```python
from build123d import *

# Parameters (mm, degrees)
F1_DEPTH = 1.06
F3_DEPTH = 1.06
F5_DEPTH = 3
F7_DEPTH = 25
F9_DEPTH = 3.6


with BuildPart() as f1:
    # F0 (on Top) → F1 (new body)
    with BuildSketch(Plane.XY):
        with BuildLine():
            ThreePointArc((-41, -6.825), (-39.256131, -8.181908), (-37.1, -8.665))
            Line((-37.1, -8.665), (-0.75, -8.665))
            ThreePointArc((-0.75, -8.665), (-0.21967, -8.44533), (0, -7.915))
            Line((0, -7.915), (0, 0))
            ThreePointArc((0, 0), (0.294358, 0.710642), (1.005, 1.005))
            Line((1.005, 1.005), (3.39, 1.005))
            Line((3.39, 1.005), (3.39, 2.125))
            ThreePointArc((3.39, 2.125), (3.097107, 2.832107), (2.39, 3.125))
            Line((2.39, 3.125), (1, 3.125))
            ThreePointArc((1, 3.125), (0.292893, 3.417893), (0, 4.125))
            Line((0, 4.125), (0, 7.915))
            ThreePointArc((0, 7.915), (-0.21967, 8.44533), (-0.75, 8.665))
            Line((-0.75, 8.665), (-37.1, 8.665))
            ThreePointArc((-37.1, 8.665), (-39.256131, 8.181908), (-41, 6.825))
            Line((-41, 6.825), (-43.4, 6.825))
            Line((-43.4, 6.825), (-43.4, 8.665))
            Line((-43.4, 8.665), (-57, 6.9))
            Line((-57, 6.9), (-57, 1.7))
            Line((-57, 1.7), (-54.7, 1.7))
            ThreePointArc((-54.7, 1.7), (-53.497918, 1.202082), (-53, 0))
            Line((-53, 0), (-53, -7.285))
            Line((-53, -7.285), (-43.4, -8.665))
            Line((-43.4, -8.665), (-43.4, -6.825))
            Line((-43.4, -6.825), (-41, -6.825))
        make_face()
    extrude(amount=-F1_DEPTH)

    # F2 (on face) → F3 (join)
    with BuildSketch(Plane.XY):
        with BuildLine():
            ThreePointArc((0, 7.915), (-0.21967, 8.44533), (-0.75, 8.665))
            Line((-0.75, 8.665), (-37.1, 8.665))
            ThreePointArc((-37.1, 8.665), (-39.256131, 8.181908), (-41, 6.825))
            Line((-41, 6.825), (-43.4, 6.825))
            Line((-43.4, 6.825), (-43.4, 8.665))
            Line((-43.4, 8.665), (-53, 7.419118))
            Line((-53, 7.419118), (-53, 0))
            ThreePointArc((-53, 0), (-53.497918, -1.202082), (-54.7, -1.7))
            Line((-54.7, -1.7), (-57, -1.7))
            Line((-57, -1.7), (-57, -6.9))
            Line((-57, -6.9), (-43.4, -8.665))
            Line((-43.4, -8.665), (-43.4, -6.825))
            Line((-43.4, -6.825), (-41, -6.825))
            ThreePointArc((-41, -6.825), (-39.256131, -8.181908), (-37.1, -8.665))
            Line((-37.1, -8.665), (-0.75, -8.665))
            ThreePointArc((-0.75, -8.665), (-0.21967, -8.44533), (0, -7.915))
            Line((0, -7.915), (0, -4.125))
            ThreePointArc((0, -4.125), (0.292893, -3.417893), (1, -3.125))
            Line((1, -3.125), (2.39, -3.125))
            ThreePointArc((2.39, -3.125), (3.097107, -2.832107), (3.39, -2.125))
            Line((3.39, -2.125), (3.39, -1.005))
            Line((3.39, -1.005), (1.005, -1.005))
            ThreePointArc((1.005, -1.005), (0.294358, -0.710642), (0, 0))
            Line((0, 0), (0, 7.915))
        make_face()
    extrude(amount=F3_DEPTH)

    # F4 (on face) → F5 (join)
    with BuildSketch(Plane(origin=(0, 0, -1.06), x_dir=(1, 0, 0), z_dir=(0, 0, -1))):
        with BuildLine():
            Line((-29.925, 2.275), (-37.725, 2.275))
            ThreePointArc((-37.725, 2.275), (-40, 0), (-37.725, -2.275))
            Line((-37.725, -2.275), (-29.925, -2.275))
            ThreePointArc((-29.925, -2.275), (-27.65, 0), (-29.925, 2.275))
        make_face()
        with BuildLine():
            Line((-4.805, 2.275), (-12.605, 2.275))
            ThreePointArc((-12.605, 2.275), (-14.88, 0), (-12.605, -2.275))
            Line((-12.605, -2.275), (-4.805, -2.275))
            ThreePointArc((-4.805, -2.275), (-2.53, 0), (-4.805, 2.275))
        make_face()
    extrude(amount=F5_DEPTH)

    # F6 (on face) → F7 (join)
    with BuildSketch(Plane.XY.offset(1.06)):
        with BuildLine():
            Line((-30.2, 1.15), (-36.7, 1.15))
            Line((-36.7, 1.15), (-36.7, -1.15))
            Line((-36.7, -1.15), (-30.2, -1.15))
            Line((-30.2, -1.15), (-30.2, -4.0125))
            ThreePointArc((-30.2, -4.0125), (-29.98033, -4.54283), (-29.45, -4.7625))
            Line((-29.45, -4.7625), (-29.05, -4.7625))
            ThreePointArc((-29.05, -4.7625), (-28.51967, -4.54283), (-28.3, -4.0125))
            Line((-28.3, -4.0125), (-28.3, -1.15))
            Line((-28.3, -1.15), (-11.6, -1.15))
            Line((-11.6, -1.15), (-11.6, -4.0125))
            ThreePointArc((-11.6, -4.0125), (-11.38033, -4.54283), (-10.85, -4.7625))
            Line((-10.85, -4.7625), (-10.45, -4.7625))
            ThreePointArc((-10.45, -4.7625), (-9.91967, -4.54283), (-9.7, -4.0125))
            Line((-9.7, -4.0125), (-9.7, -1.15))
            Line((-9.7, -1.15), (-5.2, -1.15))
            Line((-5.2, -1.15), (-5.2, 1.15))
            Line((-5.2, 1.15), (-9.7, 1.15))
            Line((-9.7, 1.15), (-9.7, 4.0125))
            ThreePointArc((-9.7, 4.0125), (-9.91967, 4.54283), (-10.45, 4.7625))
            Line((-10.45, 4.7625), (-10.85, 4.7625))
            ThreePointArc((-10.85, 4.7625), (-11.38033, 4.54283), (-11.6, 4.0125))
            Line((-11.6, 4.0125), (-11.6, 1.15))
            Line((-11.6, 1.15), (-28.3, 1.15))
            Line((-28.3, 1.15), (-28.3, 4.0125))
            ThreePointArc((-28.3, 4.0125), (-28.51967, 4.54283), (-29.05, 4.7625))
            Line((-29.05, 4.7625), (-29.45, 4.7625))
            ThreePointArc((-29.45, 4.7625), (-29.98033, 4.54283), (-30.2, 4.0125))
            Line((-30.2, 4.0125), (-30.2, 1.15))
        make_face()
    extrude(amount=F7_DEPTH)

    # F8 (on face) → F9 (join)
    with BuildSketch(Plane.XY.offset(1.06)):
        with BuildLine():
            Line((-37.95, 1.15), (-37.95, 2.9))
            ThreePointArc((-37.95, 2.9), (-38.4382, 3.489492), (-39.108336, 3.119684))
            ThreePointArc((-39.108336, 3.119684), (-39.7, 0), (-39.108336, -3.119684))
            ThreePointArc((-39.108336, -3.119684), (-38.4382, -3.489492), (-37.95, -2.9))
            Line((-37.95, -2.9), (-37.95, -1.15))
            Line((-37.95, -1.15), (-36.7, -1.15))
            Line((-36.7, -1.15), (-36.7, 1.15))
            Line((-36.7, 1.15), (-37.95, 1.15))
        make_face()
        with BuildLine():
            Line((-5.2, -1.15), (-3.95, -1.15))
            Line((-3.95, -1.15), (-3.95, -2.9))
            ThreePointArc((-3.95, -2.9), (-3.4618, -3.489492), (-2.791664, -3.119684))
            ThreePointArc((-2.791664, -3.119684), (-2.2, 0), (-2.791664, 3.119684))
            ThreePointArc((-2.791664, 3.119684), (-3.4618, 3.489492), (-3.95, 2.9))
            Line((-3.95, 2.9), (-3.95, 1.15))
            Line((-3.95, 1.15), (-5.2, 1.15))
            Line((-5.2, 1.15), (-5.2, -1.15))
        make_face()
    extrude(amount=F9_DEPTH)


solid = f1.part
```
Geometry: final body of the model. Coordinates: model frame, mm. A direction names the side the tool comes from. Coordinates: 2 decimals unless noted, no trailing zeros. Loops run counter-clockwise (first coordinate to the right, second up) from the corner with the lowest first, then second, coordinate; pieces in that order, holes last. Notation, with made-up numbers: (-38, -33) -> (-17, -33) arc R24 ccw to (-17, -8) -> close; hole circle Ø3 at (-22, 36.25). An arc over 180 degrees is marked (long way). Use a Markdown table: item, result. Add a question column.
(1) Mould query, pull axis X, two halves, no side actions, for faces 1 (the flat face through (-57, -4.3, 0.5)), 2 (the flat face through (1.7, 3.125, -0.5)), 3 (the cylindrical face through (-27.65, 0.05, -2.54)). Classes: pulls with the +X half, pulls with the -X half, needs draft (parallel to the pull), parting line crosses it, or undercut.
(2) Section query C-C, the plane x = -20.5. Return loops of the section in (y, z) (3 decimals), plus the area to 3 significant figures.
(3) Section query A-A, the plane x = -36. Return loops of the section in (y, z) (3 decimals), plus the area to 3 significant figures.
(4) Line query: line 1 along X through (y, z) = (-4, 20); line 2 along X through (y, z) = (-2.25, 1.5); line 3 along X through (y, z) = (-2, 3). Output: solid intervals per line, ascending.
(5) Section query B-B, the plane z = 23.5. Return loops of the section in (x, y), plus the area to 3 significant figures.
(6) Section query D-D, the plane x = -48.5. Return loops of the section in (y, z).
(7) Access query for faces 4 (the cylindrical face through (-39.7, 0, 2.8)), 5 (the flat face through (-42, -6.825, 0)), 6 (the cylindrical face through (-3.45, 3.49, 2.83)), 7 (the flat face through (-36.7, 0, 15)), 8 (the flat face through (-42, 6.825, 0)). Directions: +Z, -Z, +X, -X, +Y, -Y. A direction counts if a zero-diameter tool reaches every point of the face in a straight line with its end or side. Return the directions, or none.
(8) Pin query (flat end, axial travel): pin 1 Ø1.4 at (y, z) = (-3.5, 14) entering from -X; pin 2 Ø1.2 at (y, z) = (0, 14.5) entering from +X; pin 3 Ø0.6 at (y, z) = (-4.5, 0.5) entering from +X. Return the tip coordinate at first contact, or that it passes through.
Answer:
| question | item | result |
|---|---|---|
| 1 | face 1 | pulls with the -X half |
| 1 | face 2 | needs draft |
| 1 | face 3 | undercut |
| 2 | outline | (-8.665, -1.06) -> (8.665, -1.06) -> (8.665, 1.06) -> (1.15, 1.06) -> (1.15, 26.06) -> (-1.15, 26.06) -> (-1.15, 1.06) -> (-8.665, 1.06) -> close |
| 2 | area | 94.2 mm^2 |
| 3 | outline | (-8.665, -1.06) -> (-2.275, -1.06) -> (-2.275, -4.06) -> (2.275, -4.06) -> (2.275, -1.06) -> (8.665, -1.06) -> (8.665, 1.06) -> (1.15, 1.06) -> (1.15, 26.06) -> (-1.15, 26.06) -> (-1.15, 1.06) -> (-8.665, 1.06) -> close |
| 3 | area | 108 mm^2 |
| 4 | line 1 | x = -30.2 to -28.3, -11.6 to -9.7 |
| 4 | line 2 | x = -39.4 to -37.95, -30.2 to -28.3, -11.6 to -9.7, -3.95 to -2.5 |
| 4 | line 3 | x = -39.46 to -37.95, -30.2 to -28.3, -11.6 to -9.7, -3.95 to -2.44 |
| 5 | outline | (-36.7, -1.15) -> (-30.2, -1.15) -> (-30.2, -4.01) arc R0.75 ccw to (-29.45, -4.76) -> (-29.05, -4.76) arc R0.75 ccw to (-28.3, -4.01) -> (-28.3, -1.15) -> (-11.6, -1.15) -> (-11.6, -4.01) arc R0.75 ccw to (-10.85, -4.76) -> (-10.45, -4.76) arc R0.75 ccw to (-9.7, -4.01) -> (-9.7, -1.15) -> (-5.2, -1.15) -> (-5.2, 1.15) -> (-9.7, 1.15) -> (-9.7, 4.01) arc R0.75 ccw to (-10.45, 4.76) -> (-10.85, 4.76) arc R0.75 ccw to (-11.6, 4.01) -> (-11.6, 1.15) -> (-28.3, 1.15) -> (-28.3, 4.01) arc R0.75 ccw to (-29.05, 4.76) -> (-29.45, 4.76) arc R0.75 ccw to (-30.2, 4.01) -> (-30.2, 1.15) -> (-36.7, 1.15) -> close |
| 5 | area | 98.9 mm^2 |
| 6 | outline | (-8, 0) -> (-7.93, 0) -> (-7.93, -1.06) -> (8, -1.06) -> (8, 1.06) -> (-8, 1.06) -> close |
| 7 | face 4 | +Z, -X |
| 7 | face 5 | +Z, -Z, -Y |
| 7 | face 6 | +Z, +Y |
| 7 | face 7 | +Z, -X, +Y, -Y |
| 7 | face 8 | +Z, -Z, +Y |
| 8 | pin 1 | stops at x = -30.2 |
| 8 | pin 2 | stops at x = -5.2 |
| 8 | pin 3 | stops at x = 0 |
